Geometry check sheet. Reference: drawing and pictorial views, mm from the part's lowest x, y, z. A direction names the side the tool comes from. Give positions to 0.01 mm unless a question says otherwise; leave off trailing zeros. Order: outer loops, then holes, each group sorted by start corner. A loop starts at its lowest first (then second) coordinate and runs counter-clockwise, first axis right, second up.
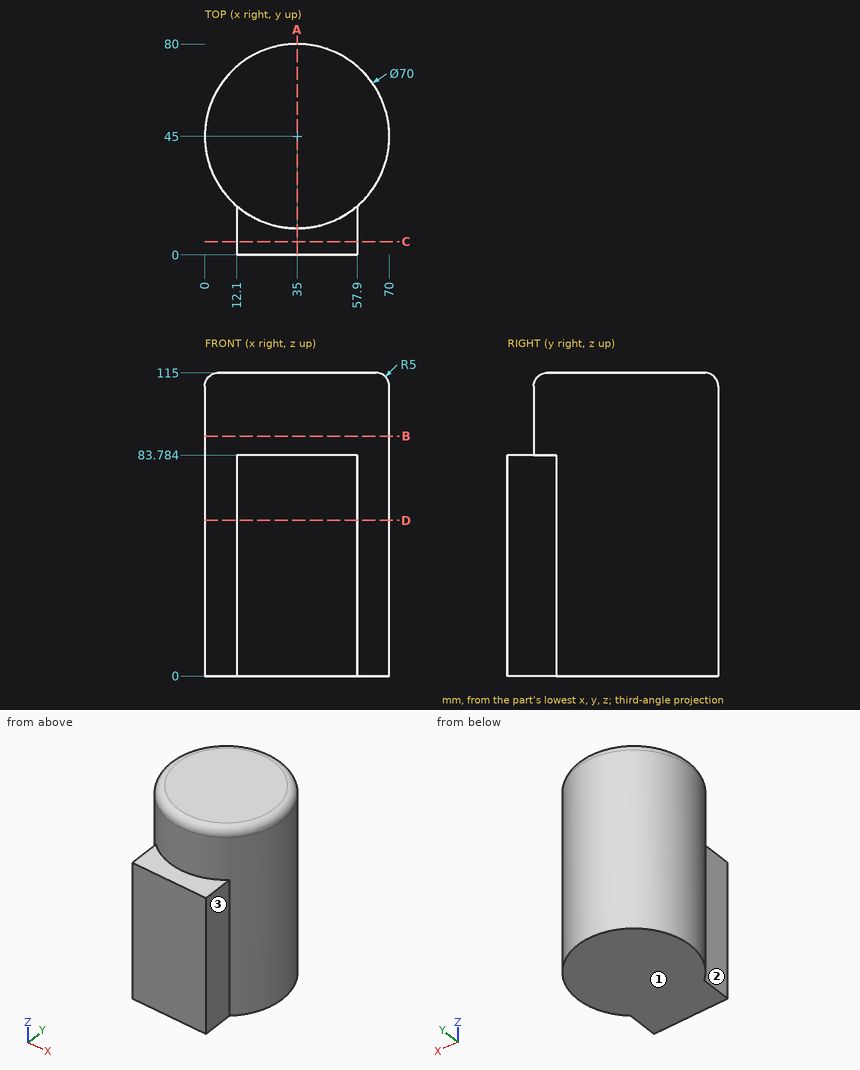
(1) Sectioned sample at B-B (z = 91). Enter the section's corners in (x, y), plus the area to 3 significant figures.
(2) Sectioned sample at A-A (x = 35). Enter the section's corners in (y, z).
(3) Tool access check on the marked faces 1, 2 and 3. Record the directions out of +Z, -Z, +X, -X, +Y, -Y that give a thin tool (end or side, any length) a straight path to the whole face; none if there is none.
(4) Sectioned sample at D-D (z = 59). Enter the section's corners in (x, y).
(5) Thickness scan on L1, parallel to X at y = 15, z = 49; L2, parallel to Z at x = 25.5, y = 11; L3, parallel to Y at x = 34.5, z = 65.5. Record the ranges inside material, lowest first.
(6) Sectioned sample at C-C (y = 5). Enter the section's corners in (x, z).
(7) Go/stop test with flat-tipped pins: P1, Ø12, axis at x = 22.5, z = 62.5, coming from the +Y side; P2, Ø5, axis at y = 55, z = 61, coming from the +X side; P3, Ø1.5, axis at x = 25, z = 65.5, coming from the +Y side (1 decimal). Record where each tip stops, or that it passes through.
Values follow:
1. outline: circle Ø70 at (35, 45)
1. area: 3,850 mm2
2. outline: (0, 0) - (80, 0) - (80, 110) arc R5 ccw to (75, 115) - (15, 115) arc R5 ccw to (10, 110) - (10, 83.78) - (0, 83.78) - close
3. face 1: -Z, +X, -X, +Y, -Y
3. face 2: +Z, -Z, -X, -Y
3. face 3: +Z, -Z, +X, -Y
4. outline: (12.1, 0) - (57.9, 0) - (57.9, 18.53) arc R35 ccw (long way) to (12.1, 18.53) - close
5. L1: x = 12.1 to 57.9
5. L2: z = 0 to 83.78
5. L3: y = 0 to 80
6. outline: (12.1, 0) - (57.9, 0) - (57.9, 83.78) - (12.1, 83.78) - close
7. P1: stops at y = 79.39
7. P2: stops at x = 69.19
7. P3: stops at y = 78.8
